Autodesk Inventor part; units mm, degrees
ref_plane "YZ Plane" through (0, 0, 0) normal (1, 0, 0) x (0, 1, 0)
ref_plane "XZ Plane" through (0, 0, 0) normal (0, 1, 0) x (-1, 0, 0)
ref_plane "XY Plane" through (0, 0, 0) normal (0, 0, 1) x (1, 0, 0)
sketch "Sketch1" plane through (0, 0, 0) normal (0, 1, 0) x (-1, 0, 0)
  circle A0 centre (0, 0) radius 135
  circle A1 centre (0, 0) radius 110
  dimension "d0" = 270
  dimension "d1" = 220
extrude "Extrusion1" add sketch "Sketch1" along normal blind 55
sketch "Sketch2" plane through (0, 0, 0) normal (0, 0, 1) x (1, 0, 0)
  circle A0 centre (0, 5) radius 18
  line L0 (135, 0) -> (-135, 0)
  point P0 (0, 0)
  dimension "d4" = 36
  dimension "d5" = 5
extrude "Extrusion2" cut sketch "Sketch2" against normal through all
sketch "Sketch3" plane through (0, 0, 0) normal (0, -1, 0) x (1, 0, 0)
  circle A0 centre (0, 0) radius 140
extrude "Extrusion3" cut sketch "Sketch3" against normal blind 20
sketch "Sketch4" plane through (0, 20, 0) normal (0, -1, 0) x (1, 0, 0)
  line L0 (0, 0) -> (70, 0)
  line L1 (80, -100) -> (60, -100)
  line L2 (60, -100) -> (60, 100)
  line L3 (60, 100) -> (80, 100)
  line L4 (80, 100) -> (80, -100)
  line L5 (80, -100) -> (60, 100) construction
  line L6 (60, -100) -> (80, 100) construction
  dimension "d10" = 70
  dimension "d11" = 20
  dimension "d12" = 200
extrude "Extrusion4" cut sketch "Sketch4" against normal through all
sketch "Sketch5" plane through (0, 55, 0) normal (0, 1, 0) x (1, 0, 0)
  circle A0 centre (0, 0) radius 127.5
  circle A1 centre (127.5, 0) radius 2
  circle A2 centre (103.1497, 74.9426) radius 2
  circle A3 centre (39.3997, 121.2597) radius 2
  circle A4 centre (-39.3997, 121.2597) radius 2
  circle A5 centre (-103.1497, 74.9426) radius 2
  circle A6 centre (-127.5, 0) radius 2
  circle A7 centre (-103.1497, -74.9426) radius 2
  circle A8 centre (-39.3997, -121.2597) radius 2
  circle A9 centre (39.3997, -121.2597) radius 2
  circle A10 centre (103.1497, -74.9426) radius 2
  dimension "d15" = 255
  dimension "d16" = 4
  dimension "d19" = 360
hole "Hole1" at (127.5, 55, 0) at (103.1497, 55, 74.9426) at (39.3997, 55, 121.2597) at (-39.3997, 55, 121.2597) at (-103.1497, 55, 74.9426) at (-127.5, 55, 0) at (-103.1497, 55, -74.9426) at (-39.3997, 55, -121.2597) at (39.3997, 55, -121.2597) at (103.1497, 55, -74.9426) direction (0, -1, 0) diameter 5 end through all
sketch "Sketch6" plane through (0, 55, 0) normal (0, 1, 0) x (1, 0, 0)
  circle A0 centre (0, 0) radius 140
extrude "Extrusion5" cut sketch "Sketch6" against normal blind 15
sketch "Sketch7" plane through (0, 40, 0) normal (0, 1, 0) x (1, 0, 0)
  circle A0 centre (0, 0) radius 140
  line L0 (80, -100) -> (80, -75.4983)
  line L1 (80, -100) -> (80, -75.4983)
  line L2 (60, -100) -> (80, -100)
  line L3 (80, -100) -> (60, -100)
  line L4 (60, -100) -> (60, -92.1954)
  line L5 (60, 100) -> (60, 92.1954)
  line L6 (60, 92.1954) -> (60, 100)
  line L7 (60, 100) -> (80, 100)
  line L8 (80, 100) -> (80, 75.4983)
  arc A1 (80, -75.4983) -> (80, 75.4983) centre (0, 0) ccw
  arc A2 (60, 92.1954) -> (60, -92.1954) centre (0, 0) ccw
  arc A3 (-25, -65) -> (25, -65) centre (0, -65) ccw
  arc A4 (25, 65) -> (-25, 65) centre (0, 65) ccw
  arc A5 (25, -27.9508) -> (25, 27.9508) centre (0, 0) ccw
  arc A6 (-25, 27.9508) -> (-25, -27.9508) centre (0, 0) ccw
  line L9 (25, 65) -> (25, 27.9508)
  line L10 (25, -27.9508) -> (25, -65)
  line L11 (-25, -65) -> (-25, -27.9508)
  line L12 (-25, 27.9508) -> (-25, 65)
extrude "Extrusion6" add sketch "Sketch7" against normal blind 1 contours L2 L4 A2 L5 L7 L8 A1 L0
sketch "Sketch8" plane through (0, 39, 0) normal (0, -1, 0) x (1, 0, 0)
  line L0 (80, -75.4983) -> (80, -100)
  line L1 (80, -100) -> (60, -100)
  line L2 (60, -100) -> (60, 100)
  line L3 (60, 100) -> (80, 100)
  line L4 (80, 100) -> (80, 75.4983)
  line L5 (80, -75.4983) -> (80, -100)
  arc A0 (80, -75.4983) -> (80, 75.4983) centre (0, 0) ccw
  arc A1 (60, 92.1954) -> (60, -92.1954) centre (0, 0) ccw
extrude "Extrusion7" add sketch "Sketch8" along normal blind 14 contours L0 L1 L2 L3 L4 A0
sketch "Sketch9" plane through (0, 20, 0) normal (0, -1, 0) x (1, 0, 0)
  arc A0 (9.9499, -134.6328) -> (-9.9499, -134.6328) centre (0, 0) ccw
  spline S0 degree 7 poles (9.9499, -134.6328) (9.4556, -134.6694) (8.9421, -134.7052) (8.4096, -134.74) (7.8582, -134.7735) (7.2882, -134.8052) (6.6998, -134.835) (5.2633, -134.8999) (4.3998, -134.933) (3.5087, -134.9604) (2.5962, -134.9814) (1.6691, -134.9951) (0.7345, -135.0012) (-1.7136, -134.9976) (-3.2083, -134.9756) (-4.6621, -134.9347) (-6.0536, -134.8776) (-7.364, -134.8084) (-8.5782, -134.7318) (-9.7236, -134.6494) (-9.7616, -134.6466) (-9.7995, -134.6439) (-9.8372, -134.6411) (-9.8749, -134.6384) (-9.9124, -134.6356) (-9.9499, -134.6328) knots 0 0 0 0 0 0 0 0 0.214533 0.214533 0.214533 0.214533 0.214533 0.214533 0.508291 0.508291 0.508291 0.508291 0.508291 0.508291 0.983641 0.983641 0.983641 0.983641 0.983641 0.983641 1 1 1 1 1 1 1 1
  line L0 (0, 135) -> (0, -135)
  line L1 (132.949, -23.4425) -> (-132.949, 23.4425)
  point P0 (0, 0)
  dimension "d40" = 80
extrude "Extrusion8" cut sketch "Sketch9" against normal through all contours S0 L0 L1 A0 | L1 L0 A0 | S0 A0 L1 L0 picked at (5.2242, 89.6957)
sketch "Sketch10" plane through (-132.949, 20, 23.4425) normal (-0.1736482, 0, -0.9848078) x (-0.9848078, 0, 0.1736482)
  line L0 (-111.5575, 20) -> (0, 20)
  line L1 (-2.5, 20) -> (15, 20)
  line L2 (20, 15) -> (20, 5)
  line L3 (15, 0) -> (-2.5, 0)
  line L4 (-2.5, 0) -> (-2.5, 20)
  line L5 (0, 20) -> (0, 0)
  arc A0 (20, 15) -> (15, 20) centre (15, 15) ccw
  arc A1 (15, 0) -> (20, 5) centre (15, 5) ccw
  point P0 (-135, -20)
  point P1 (20, 0)
  point P2 (20, 20)
  dimension "d43" = 22.5
  dimension "d44" = 20
  dimension "d45" = 20
  dimension "d46" = 5
extrude "Extrusion9" add sketch "Sketch10" against normal blind 10
sketch "Sketch11" plane through (0, 20, 135) normal (1, 0, 0) x (0, 0, -1)
  line L0 (2.5, 20.0082) -> (-15, 20.0082)
  line L1 (-20, 15.0082) -> (-20, 5.0082)
  line L2 (-15, 0.0082) -> (2.5, 0.0082)
  line L3 (2.5, 0.0082) -> (2.5, 20.0082)
  line L4 (0, 0) -> (0, 20)
  arc A0 (-15, 20.0082) -> (-20, 15.0082) centre (-15, 15.0082) ccw
  arc A1 (-20, 5.0082) -> (-15, 0.0082) centre (-15, 5.0082) ccw
  point P0 (135, -20)
  point P1 (-20, 0.0082)
  point P2 (-20, 20.0082)
  dimension "d50" = 22.5
  dimension "d51" = 20
  dimension "d52" = 20
  dimension "d53" = 5
extrude "Extrusion10" add sketch "Sketch11" against normal blind 10
sketch "Sketch12" plane through (-131.2126, 20, 33.2906) normal (0.1736482, 0, 0.9848078) x (0.9848078, 0, -0.1736482)
  line L0 (-15, 0) -> (0.3709, 0)
  line L1 (-20, 15) -> (-20, 5)
  point P0 (135, -20)
  point P1 (-10, 10)
  dimension "d58" = 10
  dimension "d59" = 10
hole "Hole2" at (-141.0606, 30, 35.0271) direction (-0.1736482, 0, -0.9848078) diameter 8.2 end through all counterbore diameter 13.2 counterbore depth 6
sketch "Sketch13" plane through (-10, 20, 135) normal (-1, 0, 0) x (0, 0, 1)
  line L0 (7.2662, 3.4082) -> (3.4, 7.2743)
  line L1 (3.4, 7.2743) -> (3.4, 12.742)
  line L2 (3.4, 12.742) -> (7.2662, 16.6082)
  line L3 (7.2662, 16.6082) -> (12.7338, 16.6082)
  line L4 (12.7338, 16.6082) -> (16.6, 12.742)
  line L5 (16.6, 12.742) -> (16.6, 7.2743)
  line L6 (16.6, 7.2743) -> (12.7338, 3.4082)
  line L7 (12.7338, 3.4082) -> (7.2662, 3.4082)
  line L8 (-0.3709, 0.0082) -> (15, 0.0082)
  line L9 (20, 5.0082) -> (20, 15.0082)
  point P0 (-135, -20)
  point P1 (10, 10.0082)
  dimension "d67" = 10
  dimension "d68" = 10
  dimension "d69" = 13.2
extrude "Extrusion11" cut sketch "Sketch13" against normal blind 6
sketch "Sketch14" plane through (-4, 20, 135) normal (-1, 0, 0) x (0, 0, 1)
  line L0 (15, 0.0082) -> (0, 0.0082)
  line L1 (20, 15.0082) -> (20, 5.0082)
  point P0 (-135, -20)
  point P1 (10, 10.0082)
  dimension "d72" = 10
  dimension "d73" = 10
hole "Hole3" at (-4, 30.0082, 145) direction (1, 0, 0) diameter 8.2 end through all
properties part number "Cylinder Spacer Top_Q4"
For this review, take the finished solid that the model builds, in its own axes (mm). A direction names the side the tool comes from. Give positions to 0.01 mm unless a question says otherwise; leave off trailing zeros. Write each loop counter-clockwise with the first axis right and the second up, starting at its lowest first coordinate (ties: lowest second). Pieces come first, ordered by that corner, then holes.
Item 1: Insertion check: P1, Ø8, axis at x = -6.5, z = 139, coming from the -Y side; P2, Ø0.8, axis at y = 39.5, z = 42.5, coming from the +X side; P3, Ø10, axis at y = 32.5, z = 144.5, coming from the -X side. Each pin has a flat end and moves straight along its axis. Give the tip position at first contact, or say it passes through.
Item 2: Machinability: for faces 4 (the face through (-7.042, 25.368, 149.694)), 5 (the face through (-69.88, 29.37, 84.95)), 6 (the face through (-4.93, 38.58, 153.5)), which of the approach directions +Z, -Z, +X, -X, +Y, -Y give a long, thin tool a straight path to every point of the face, cutting with its end or side? Answer none if there is none.
Item 3: The part is to be moulded in two halves that separate along Y. For faces 1 (the face through (-5, 30, 155)), 2 (the face through (-7, 23.408, 145)), 3 (the face through (-4.93, 21.51, 153.57)), say which applies: +Y half, -Y half, draft (parallel to the pull), parting line (faces both ways), or undercut.
Item 4: Take a section at A-A (z = 145). Give the boundary of the cut face in (x, y), and give its area (3 significant figures).
Item 5: Wall thickness on probe 1 along Y at (x, z) = (-1, 145); probe 2 along X at (y, z) = (21.25, 138.5); probe 3 along Z at (x, y) = (-102, 24): over which ranges is each line inside the solid? List them lowest first.
Item 6: Take a section at C-C (z = 39.5). Give the boundary of the cut face in (x, y), and give its area (3 significant figures).
Item 7: Take a section at B-B (x = -67.5). Give the boundary of the cut face in (y, z), and give its area (3 significant figures).
Item 8: Take a section at D-D (z = 128). Give the boundary of the cut face in (x, y), and give its area (3 significant figures).
Established:
1. P1: stops at y = 20.01
1. P2: stops at x = -25
1. P3: stops at x = -10
2. face 4: -X
2. face 5: -Z, +X, -Y
2. face 6: +Z, +X, -X, +Y
3. face 1: draft
3. face 2: undercut
3. face 3: -Y half
4. outline: (-10, 20.01) - (0, 20.01) - (0, 25.91) - (-4, 25.91) - (-4, 23.41) - (-10, 23.41) - close; (-10, 36.61) - (-4, 36.61) - (-4, 34.11) - (0, 34.11) - (0, 40.01) - (-10, 40.01) - close
4. area: 88.0 mm2
5. probe 1: y = 20.01 to 25.91, 34.11 to 40.01
5. probe 2: x = -10 to 0
5. probe 3: z = 41.18 to 72.72, 77.16 to 88.44
6. outline: (-129.09, 20) - (-102.66, 20) - (-102.66, 39) - (-25, 39) - (-25, 40) - (-129.09, 40) - close
6. area: 606 mm2
7. outline: (20, 86.85) - (39, 86.85) - (39, 11.9) - (40, 11.9) - (40, 116.91) - (20, 116.91) - close
7. area: 676 mm2
8. outline: (-42.91, 20) - (0, 20) - (0, 40) - (-42.91, 40) - close
8. area: 858 mm2
